Read the model definition and answer for the solid it produces. Units are mm, in the model's axes. A direction names the side the tool comes from. Give positions to 0.01 mm unless a question says otherwise; leave off trailing zeros. Loops run counter-clockwise (first coordinate to the right, second up) from the corner with the lowest first, then second, coordinate; pieces in that order, holes last. Notation, with made-up numbers: (-12.5, 41) - (-8.5, 41) arc R15 cw to (-8.5, 67) - close; hole circle Ø6 at (59.5, 44). An arc over 180 degrees is marked (long way). Put each result on its own line as item: value. Start each with the question number.
1. Given pin 1 Ø5 at (y, z) = (-52, -15.5) entering from +X; pin 2 Ø3 at (y, z) = (-11.5, -24.5) entering from -X; pin 3 Ø6 at (y, z) = (-53.5, -57) entering from -X; pin 4 Ø10 at (x, z) = (38, -89.5) entering from -Y, each flat-ended and moving along its own axis, determine where each tip first touches the part or whether it passes through.
2. A cutting plane is placed at B-B, the plane x = 0. Determine the outline of the cut face in (y, z).
3. For a pull along Z with two mould halves and no side action, classify faces 3 (the flat face through (27, -25.4, -20)), 4 (the flat face through (-0.7, -88.9, -17.6)), 5 (the cylindrical face through (-15.259, -45.072, -2.346)) as released by +Z, released by -Z, zero draft, split by the parting line, or undercut.
4. A cutting plane is placed at C-C, the plane y = -78. Determine the outline of the cut face in (x, z).
5. A cutting plane is placed at D-D, the plane y = -65. Determine the outline of the cut face in (x, z), plus the area to 3 significant figures.
6. Consider L1, parallel to Z at x = 0, y = -84; L2, parallel to X at y = -3.75, z = -50.8; L3, parallel to X at y = -58.5, z = -50.8. Determine where each line is inside the solid, lowest interval first. Write a range as from..to.
7. For faces 1 (the cylindrical face through (-30.9, -21.3, -84.5)), 2 (the flat face through (-19, 0, -9)), determine the directions among +Z, -Z, +X, -X, +Y, -Y from which every point of the face is accessible in a straight line to the end or side of a thin tool.
8. A cutting plane is placed at A-A, the plane z = -50.8. Determine the outline of the cut face in (x, y).
```python
from build123d import *


with BuildPart() as part:
    # Sketch1 → Revolve1 (revolve)
    with BuildSketch(Plane(origin=(0, 0, 0), x_dir=(0, 0, -1), z_dir=(1, 0, 0))):
        with BuildLine():
            Line((0, 0), (0, -88.9))
            Line((0, -88.9), (10.16, -88.9))
            Line((10.16, -88.9), (17.78, -88.9))
            Line((17.78, -88.9), (17.78, -76.2))
            Line((17.78, -76.2), (10.16, -76.2))
            Line((10.16, -76.2), (10.16, -25.4))
            Line((10.16, -25.4), (5.08, -25.4))
            Line((5.08, -25.4), (5.08, -17.355896906))
            ThreePointArc((5.08, -17.355896906), (2.032, -12.7), (5.08, -8.044103094))
            Line((5.08, -8.044103094), (5.08, 0))
            Line((5.08, 0), (0, 0))
        make_face()
    revolve(axis=Axis((0, -28.313229254, -50.8), (0, -1, 0)))


solid = part.part
```
Return value:
1. pin 1: stops at x = 38.79
1. pin 2: stops at x = -44.34
1. pin 3: stops at x = -50.7
1. pin 4: stops at y = -88.9
2. outline: (-88.9, -101.6) - (0, -101.6) - (0, -96.52) - (-8.04, -96.52) arc R5.08 cw to (-17.36, -96.52) - (-25.4, -96.52) - (-25.4, -91.44) - (-76.2, -91.44) - (-76.2, -83.82) - (-88.9, -83.82) - close; (-88.9, -17.78) - (-76.2, -17.78) - (-76.2, -10.16) - (-25.4, -10.16) - (-25.4, -5.08) - (-17.36, -5.08) arc R5.08 cw to (-8.04, -5.08) - (0, -5.08) - (0, 0) - (-88.9, 0) - close
3. face 3: undercut
3. face 4: zero draft
3. face 5: split by the parting line
4. outline: circle Ø101.6 at (0, -50.8); hole circle Ø66.04 at (0, -50.8)
5. outline: circle Ø101.6 at (0, -50.8); hole circle Ø81.28 at (0, -50.8)
5. area: 2,920 mm2
6. L1: z = -101.6..-83.82, -17.78..0
6. L2: x = -50.8..-45.72, 45.72..50.8
6. L3: x = -50.8..-40.64, 40.64..50.8
7. face 1: +Y
7. face 2: +Z, -Z, +X, -X, +Y
8. outline: (-50.8, -88.9) - (-33.02, -88.9) - (-33.02, -76.2) - (-40.64, -76.2) - (-40.64, -25.4) - (-45.72, -25.4) - (-45.72, -17.36) arc R5.08 cw to (-45.72, -8.04) - (-45.72, 0) - (-50.8, 0) - close; (33.02, -88.9) - (50.8, -88.9) - (50.8, 0) - (45.72, 0) - (45.72, -8.04) arc R5.08 cw to (45.72, -17.36) - (45.72, -25.4) - (40.64, -25.4) - (40.64, -76.2) - (33.02, -76.2) - close
